Geometry: final body of the model. Coordinates: model frame, mm. A direction names the side the tool comes from. Give positions to 0.01 mm unless a question says otherwise; leave off trailing zeros. Write each loop counter-clockwise with the first axis right and the second up, starting at its lowest first coordinate (ties: lowest second). Pieces come first, ordered by that corner, then holes. Notation, with made-up numbers: (62.25, 36) - (91.25, 36) arc R22 cw to (91.25, 74) - close; hole circle Ø9 at (43, 81). An arc over 180 degrees is marked (long way). Return JSON: item names as keys, results as strings.
from build123d import *

# Parameters (mm, degrees)
SKETCH1_R           = 3.45
BOSS_EXTRUDE1_DEPTH = 1.5


with BuildPart() as part:
    # Sketch1 → Boss-Extrude1 (new, symmetric)
    with BuildSketch(Plane(origin=(0, 0, 0), x_dir=(1, 0, 0), z_dir=(0, 1, 0))):
        with BuildLine():
            Line((19.451315789, 3.470780036), (0.767236842, 5.900326061))
            ThreePointArc((0.767236842, 5.900326061), (-5.95, 0), (0.767236842, -5.900326061))
            Line((0.767236842, -5.900326061), (19.451315789, -3.470780036))
            ThreePointArc((19.451315789, -3.470780036), (22.5, 0), (19.451315789, 3.470780036))
        make_face()
        with Locations(Location((0, 0, 0), (0, 0, 270))):
            Circle(SKETCH1_R, mode=Mode.SUBTRACT)
        with BuildLine():
            Line((19, -1.5), (17, -1.5))
            ThreePointArc((17, -1.5), (15.5, 0), (17, 1.5))
            Line((17, 1.5), (19, 1.5))
            ThreePointArc((19, 1.5), (20.5, 0), (19, -1.5))
        make_face(mode=Mode.SUBTRACT)
    extrude(amount=BOSS_EXTRUDE1_DEPTH, both=True)


solid = part.part
Q1. Set-up query: faces 4 (the flat face through (10.24, 0.02, -4.67)), 5 (the flat face through (18, 0, 1.5)). Return all of +Z, -Z, +X, -X, +Y, -Y with unobstructed straight access to the full face (end or side cutting, diameter ignored); none if empty.
Answer key:
{"face 4": "-Z, +X, +Y, -Y", "face 5": "+Y, -Y"}
Q2. Section query A-A, the plane x = 0. Return the cut outline in (y, z).
Answer key:
{"outline": "(-1.5, -5.95) - (1.5, -5.95) - (1.5, -3.45) - (-1.5, -3.45) - close; (-1.5, 3.45) - (1.5, 3.45) - (1.5, 5.95) - (-1.5, 5.95) - close"}
Q3. Mould query, pull axis Z, two halves, no side actions, for faces 1 (the flat face through (18, 0, -1.5)), 2 (the flat face through (8, -1.5, 0)), 3 (the flat face through (10, 0, 4.7)). Classes: pulls with the +Z half, pulls with the -Z half, needs draft (parallel to the pull), parting line crosses it, or undercut.
Answer key:
{"face 1": "undercut", "face 2": "needs draft", "face 3": "pulls with the +Z half"}
Q4. Material intervals for probe 1 along X at (y, z) = (-0.2, 0); probe 2 along X at (y, z) = (1, -2); probe 3 along Z at (x, y) = (20.75, -0.8), sorted ascending. Write a range as [from, to].
Answer key:
{"probe 1": "x = [-5.95, -3.45], [3.45, 15.5], [20.5, 22.5]", "probe 2": "x = [-5.6, -2.81], [2.81, 21.87]", "probe 3": "z = [-3.03, 3.03]"}
Q5. Pin query (flat end, axial travel): P1, Ø1, axis at x = 18, y = 0.5, coming from the +Z side; P2, Ø1.5, axis at x = 17, y = 1, coming from the +Z side; P3, Ø1, axis at x = 18, y = -0.5, coming from the -Z side. Return the tip coordinate at first contact, or that it passes through.
Answer key:
{"P1": "stops at z = 3.72", "P2": "stops at z = 3.89", "P3": "stops at z = -3.72"}
Q6. Section query B-B, the plane z = 0. Return the cut outline in (x, y).
Answer key:
{"outline": "(-5.95, -1.5) - (-3.45, -1.5) - (-3.45, 1.5) - (-5.95, 1.5) - close; (3.45, -1.5) - (15.5, -1.5) - (15.5, 1.5) - (3.45, 1.5) - close; (20.5, -1.5) - (22.5, -1.5) - (22.5, 1.5) - (20.5, 1.5) - close"}
Q7. Section query C-C, the plane y = 0.95. Return the cut outline in (x, z), plus the area to 3 significant figures.
Answer key:
{"outline": "(0.77, -5.9) - (19.45, -3.47) arc R3.5 ccw to (19.45, 3.47) - (0.77, 5.9) arc R5.95 ccw (long way) to start; hole circle Ø6.9 at (0, 0); hole (17, -1.5) - (19, -1.5) arc R1.5 ccw to (19, 1.5) - (17, 1.5) arc R1.5 ccw to start", "area": "205 mm^2"}
Q8. Section query D-D, the plane z = 1.75. Return the cut outline in (x, y).
Answer key:
{"outline": "(-5.69, -1.5) - (-2.97, -1.5) - (-2.97, 1.5) - (-5.69, 1.5) - close; (2.97, -1.5) - (22.03, -1.5) - (22.03, 1.5) - (2.97, 1.5) - close"}
